Work out the finished part from the listing and answer in its coordinate system (mm). Round coordinates to 2 decimals unless told otherwise and drop trailing zeros. Use one line per item in the form item = value. Start each with the question number.
Q1. For a pull along X with two mould halves and no side action, classify faces 1 (the flat face through (-10, -6, -148)), 2 (the flat face through (10, 6, -148)), 3 (the flat face through (6, -10, -148)) as +X half, -X half, draft (parallel to the pull), parting line (faces both ways), or undercut.
Q2. Find the intervals of material crossed by line 1 (Y direction, x = -3.5, z = -258.5); line 2 (Y direction, x = 0, z = -140); line 3 (X direction, y = 4.5, z = -174), in increasing order. Write a range as [from, to].
Q3. Given P1, Ø1.3, axis at x = 0, z = -134, coming from the -Y side; P2, Ø1.3, axis at y = -0.5, z = -219, coming from the +X side; P3, Ø1.5, axis at x = -1.5, z = -89.5, coming from the -Y side, each flat-ended and moving along its own axis, determine where each tip first touches the part or whether it passes through.
from build123d import *

# Parameters (mm, degrees)
SKETCH2_R           = 2.05
BOSS_EXTRUDE1_DEPTH = 300


with BuildPart() as part:
    # Sketch2 → Boss-Extrude1 (new body)
    with BuildSketch(Plane.XY):
        with BuildLine():
            Line((-3.642230561, 1.287773026), (-3.642230561, -1.287773026))
            ThreePointArc((-3.642230561, -1.287773026), (-3.87999308, -2.483085929), (-4.55708345, -3.496423279))
            Line((-4.55708345, -3.496423279), (-7.182004606, -6.121344434))
            ThreePointArc((-7.182004606, -6.121344434), (-7.704200045, -6.225215565), (-8, -5.782519648))
            Line((-8, -5.782519648), (-8, -3.622007668))
            ThreePointArc((-8, -3.622007668), (-8.161974206, -3.230967343), (-8.553014531, -3.068993137))
            Line((-8.553014531, -3.068993137), (-9.443284204, -3.068993137))
            ThreePointArc((-9.443284204, -3.068993137), (-9.836715763, -3.229656566), (-10, -3.622007668))
            Line((-10, -3.622007668), (-10, -8.939033256))
            ThreePointArc((-10, -8.939033256), (-9.689250035, -9.689250035), (-8.939033256, -10))
            Line((-8.939033256, -10), (-3.622007668, -10))
            ThreePointArc((-3.622007668, -10), (-3.229656566, -9.836715763), (-3.068993137, -9.443284204))
            Line((-3.068993137, -9.443284204), (-3.068993137, -8.553014531))
            ThreePointArc((-3.068993137, -8.553014531), (-3.230967343, -8.161974206), (-3.622007668, -8))
            Line((-3.622007668, -8), (-5.782519648, -8))
            ThreePointArc((-5.782519648, -8), (-6.225215565, -7.704200045), (-6.121344434, -7.182004606))
            Line((-6.121344434, -7.182004606), (-3.496423279, -4.55708345))
            ThreePointArc((-3.496423279, -4.55708345), (-2.483085929, -3.87999308), (-1.287773026, -3.642230561))
            Line((-1.287773026, -3.642230561), (1.287773026, -3.642230561))
            ThreePointArc((1.287773026, -3.642230561), (2.483085929, -3.87999308), (3.496423279, -4.55708345))
            Line((3.496423279, -4.55708345), (6.121344434, -7.182004606))
            ThreePointArc((6.121344434, -7.182004606), (6.225215565, -7.704200045), (5.782519648, -8))
            Line((5.782519648, -8), (3.622007668, -8))
            ThreePointArc((3.622007668, -8), (3.230967343, -8.161974206), (3.068993137, -8.553014531))
            Line((3.068993137, -8.553014531), (3.068993137, -9.443284204))
            ThreePointArc((3.068993137, -9.443284204), (3.229656566, -9.836715763), (3.622007668, -10))
            Line((3.622007668, -10), (8.939033256, -10))
            ThreePointArc((8.939033256, -10), (9.689250035, -9.689250035), (10, -8.939033256))
            Line((10, -8.939033256), (10, -3.622007668))
            ThreePointArc((10, -3.622007668), (9.836715763, -3.229656566), (9.443284204, -3.068993137))
            Line((9.443284204, -3.068993137), (8.553014531, -3.068993137))
            ThreePointArc((8.553014531, -3.068993137), (8.161974206, -3.230967343), (8, -3.622007668))
            Line((8, -3.622007668), (8, -5.782519648))
            ThreePointArc((8, -5.782519648), (7.704200045, -6.225215565), (7.182004606, -6.121344434))
            Line((7.182004606, -6.121344434), (4.55708345, -3.496423279))
            ThreePointArc((4.55708345, -3.496423279), (3.87999308, -2.483085929), (3.642230561, -1.287773026))
            Line((3.642230561, -1.287773026), (3.642230561, 1.287773026))
            ThreePointArc((3.642230561, 1.287773026), (3.87999308, 2.483085929), (4.55708345, 3.496423279))
            Line((4.55708345, 3.496423279), (7.182004606, 6.121344434))
            ThreePointArc((7.182004606, 6.121344434), (7.704200045, 6.225215565), (8, 5.782519648))
            Line((8, 5.782519648), (8, 3.622007668))
            ThreePointArc((8, 3.622007668), (8.161974206, 3.230967343), (8.553014531, 3.068993137))
            Line((8.553014531, 3.068993137), (9.443284204, 3.068993137))
            ThreePointArc((9.443284204, 3.068993137), (9.836715763, 3.229656566), (10, 3.622007668))
            Line((10, 3.622007668), (10, 8.939033256))
            ThreePointArc((10, 8.939033256), (9.689250035, 9.689250035), (8.939033256, 10))
            Line((8.939033256, 10), (3.622007668, 10))
            ThreePointArc((3.622007668, 10), (3.229656566, 9.836715763), (3.068993137, 9.443284204))
            Line((3.068993137, 9.443284204), (3.068993137, 8.553014531))
            ThreePointArc((3.068993137, 8.553014531), (3.230967343, 8.161974206), (3.622007668, 8))
            Line((3.622007668, 8), (5.782519648, 8))
            ThreePointArc((5.782519648, 8), (6.225215565, 7.704200045), (6.121344434, 7.182004606))
            Line((6.121344434, 7.182004606), (3.496423279, 4.55708345))
            ThreePointArc((3.496423279, 4.55708345), (2.483085929, 3.87999308), (1.287773026, 3.642230561))
            Line((1.287773026, 3.642230561), (-1.287773026, 3.642230561))
            ThreePointArc((-1.287773026, 3.642230561), (-2.483085929, 3.87999308), (-3.496423279, 4.55708345))
            Line((-3.496423279, 4.55708345), (-6.121344434, 7.182004606))
            ThreePointArc((-6.121344434, 7.182004606), (-6.225215565, 7.704200045), (-5.782519648, 8))
            Line((-5.782519648, 8), (-3.622007668, 8))
            ThreePointArc((-3.622007668, 8), (-3.230967343, 8.161974206), (-3.068993137, 8.553014531))
            Line((-3.068993137, 8.553014531), (-3.068993137, 9.443284204))
            ThreePointArc((-3.068993137, 9.443284204), (-3.229656566, 9.836715763), (-3.622007668, 10))
            Line((-3.622007668, 10), (-8.939033256, 10))
            ThreePointArc((-8.939033256, 10), (-9.689250035, 9.689250035), (-10, 8.939033256))
            Line((-10, 8.939033256), (-10, 3.622007668))
            ThreePointArc((-10, 3.622007668), (-9.836715763, 3.229656566), (-9.443284204, 3.068993137))
            Line((-9.443284204, 3.068993137), (-8.553014531, 3.068993137))
            ThreePointArc((-8.553014531, 3.068993137), (-8.161974206, 3.230967343), (-8, 3.622007668))
            Line((-8, 3.622007668), (-8, 5.782519648))
            ThreePointArc((-8, 5.782519648), (-7.704200045, 6.225215565), (-7.182004606, 6.121344434))
            Line((-7.182004606, 6.121344434), (-4.55708345, 3.496423279))
            ThreePointArc((-4.55708345, 3.496423279), (-3.87999308, 2.483085929), (-3.642230561, 1.287773026))
        make_face()
        Circle(SKETCH2_R, mode=Mode.SUBTRACT)
    extrude(amount=-BOSS_EXTRUDE1_DEPTH)


solid = part.part
Found:
q1.face_1 = -X half
q1.face_2 = +X half
q1.face_3 = draft
q2.line_1 = [-9.99, -8.01], [-4.56, 4.56], [8.01, 9.99]
q2.line_2 = [-3.64, -2.05], [2.05, 3.64]
q2.line_3 = [-10, -8], [-5.56, -3.44], [3.44, 5.56], [8, 10]
q3.P1 = -3.64
q3.P2 = 3.64
q3.P3 = -3.79
